Print and shaded views of the part. All mm, measured from the part's lowest x, y and z. A direction names the side the tool comes from. Round coordinates to 2 decimals unless told otherwise and drop trailing zeros. Write each loop counter-clockwise with the first axis right and the second up, starting at its lowest first coordinate (ties: lowest second). Pieces come first, ordered by that corner, then holes. Notation, with made-up numbers: (77.5, 49.5) - (82.5, 49.5) arc R29 ccw to (82.5, 69.5) - close; hole circle Ø8 at (-33, 83). An arc over 180 degrees is marked (long way). Answer as a JSON object with one key per item and string values. Group by question number.
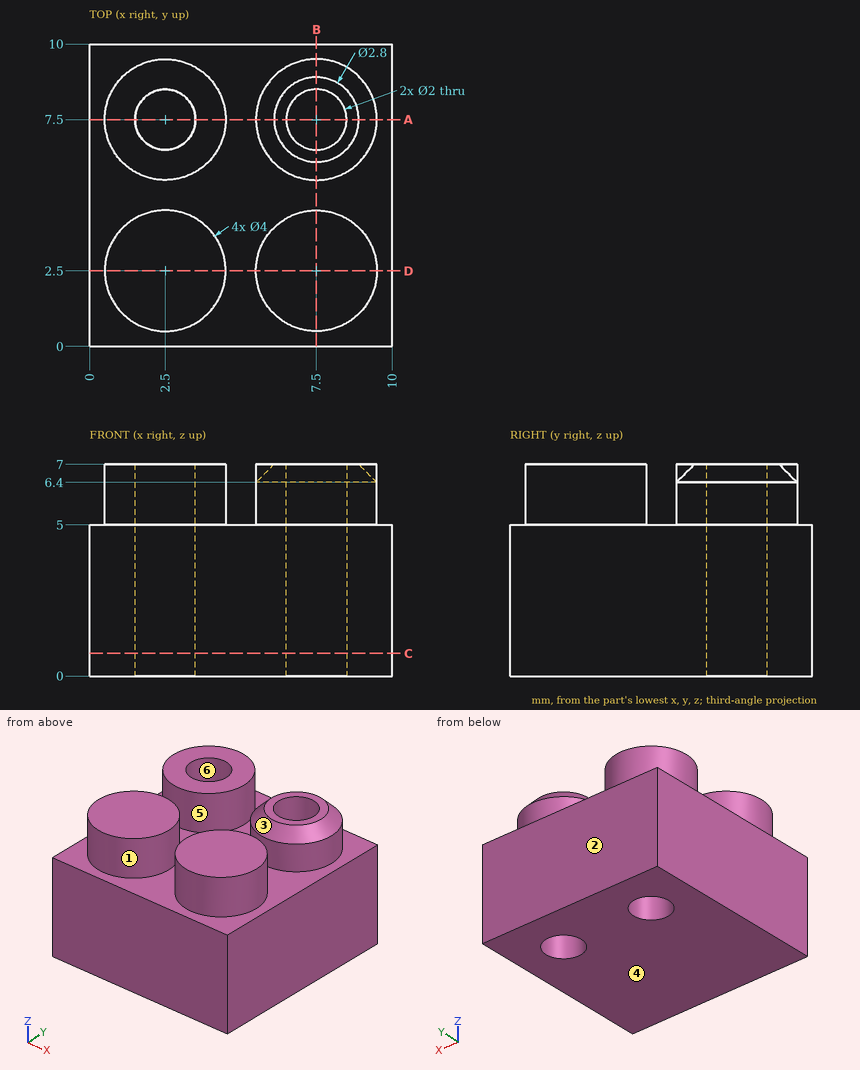
(1) Pull direction Y, two halves, no side cores. Call the marked faces 1, 2, 3 and 4: pulls with the +Y half, pulls with the -Y half, needs draft (parallel to the pull), parting line crosses it, or undercut.
(2) Slice it at C-C (z = 0.75). Write the cut outline in (x, y), then the cut area to 3 significant figures.
(3) Slice it at D-D (y = 2.5). Write the cut outline in (x, z).
(4) 3-axis set-ups, long thin cutter, end or side, ignore diameter. For the marked faces 5 and 6: which of +Z, -Z, +X, -X, +Y, -Y reach the whole face in a straight line?
(5) Flat gauge pins, fed straight in: pin 1 (1.5 mm diameter, centred on x = 3.5, y = 4.5, fed in from -Z); pin 2 (1.2 mm diameter, centred on x = 2.5, y = 7.5, fed in from +Z). Where does each tip first touch, or does it go through?
(6) Slice it at B-B (x = 7.5). Write the cut outline in (y, z), then the cut area to 3 significant figures.
(7) Drill centre lines: line 1 (Y direction, x = 7.5, z = 5.5); line 2 (Y direction, x = 7.5, z = 3.5); line 3 (X direction, y = 6.75, z = 6.25). Where is each one in solid material? Low to high. Write a range as from..to.
(8) Slice it at A-A (y = 7.5). Write the cut outline in (x, z).
Answer:
{
 "1": {"face 1": "undercut", "face 2": "pulls with the +Y half", "face 3": "undercut", "face 4": "needs draft"},
 "2": {"outline": "(0, 0) - (10, 0) - (10, 10) - (0, 10) - close; hole circle Ø2 at (2.5, 7.5); hole circle Ø2 at (7.5, 7.5)", "area": "93.7 mm²"},
 "3": {"outline": "(0, 0) - (10, 0) - (10, 5) - (9.5, 5) - (9.5, 7) - (5.5, 7) - (5.5, 5) - (4.5, 5) - (4.5, 7) - (0.5, 7) - (0.5, 5) - (0, 5) - close"},
 "4": {"face 5": "+Z", "face 6": "+Z, -Z"},
 "5": {"pin 1": "z = 0", "pin 2": "through"},
 "6": {"outline": "(0, 0) - (6.5, 0) - (6.5, 7) - (6.1, 7) - (5.5, 6.4) - (5.5, 5) - (4.5, 5) - (4.5, 7) - (0.5, 7) - (0.5, 5) - (0, 5) - close; (8.5, 0) - (10, 0) - (10, 5) - (9.5, 5) - (9.5, 6.4) - (8.9, 7) - (8.5, 7) - close", "area": "51.6 mm²"},
 "7": {"line 1": "0.5..4.5, 5.5..6.5, 8.5..9.5", "line 2": "0..6.5, 8.5..10", "line 3": "0.65..1.84, 3.16..4.35, 5.65..6.84, 8.16..9.35"},
 "8": {"outline": "(0, 0) - (1.5, 0) - (1.5, 7) - (0.5, 7) - (0.5, 5) - (0, 5) - close; (3.5, 0) - (6.5, 0) - (6.5, 7) - (6.1, 7) - (5.5, 6.4) - (5.5, 5) - (4.5, 5) - (4.5, 7) - (3.5, 7) - close; (8.5, 0) - (10, 0) - (10, 5) - (9.5, 5) - (9.5, 6.4) - (8.9, 7) - (8.5, 7) - close"}
}
